Autodesk Inventor part; units mm, degrees
ref_plane "YZ Plane" through (0, 0, 0) normal (1, 0, 0) x (0, 1, 0)
ref_plane "XZ Plane" through (0, 0, 0) normal (0, 1, 0) x (-1, 0, 0)
ref_plane "XY Plane" through (0, 0, 0) normal (0, 0, 1) x (1, 0, 0)
sketch "Sketch1" plane through (0, 0, 0) normal (0, 0, 1) x (1, 0, 0)
  line L0 (-4.5, -2.26) -> (4.5, -2.26)
  line L1 (4.5, -2.26) -> (4.5, 2.26)
  line L2 (4.5, 2.26) -> (-4.5, 2.26)
  line L3 (-4.5, 2.26) -> (-4.5, -2.26)
  line L4 (-4.5, -2.26) -> (4.5, 2.26) construction
  line L5 (4.5, -2.26) -> (-4.5, 2.26) construction
  point P0 (0, 0)
  dimension "d0" = 9
  dimension "d1" = 4.52
extrude "Extrusion1" add sketch "Sketch1" along normal blind 2.5
sketch "Sketch2" plane through (0, 0, 0) normal (0, 0, 1) x (1, 0, 0)
  line L0 (-6, -5) -> (6, -5)
  line L1 (6, -5) -> (6, 5)
  line L2 (6, 5) -> (-6, 5)
  line L3 (-6, 5) -> (-6, -5)
  line L4 (-6, -5) -> (6, 5) construction
  line L5 (6, -5) -> (-6, 5) construction
  point P0 (0, 0)
  dimension "d4" = 12
  dimension "d5" = 10
extrude "Extrusion2" add sketch "Sketch2" against normal blind 20
fillet "Fillet1" radius 2 4 edges at (-6, 5, -10) (6, 5, -10) (6, -5, -10) (-6, -5, -10)
sketch "Sketch3" plane through (0, 0, 0) normal (0, 0, 1) x (1, 0, 0)
  line L0 (-9, 0) -> (9, 0) construction
  circle A0 centre (-9, 0) radius 4.05
  circle A1 centre (9, 0) radius 4.05
  line L1 (-9, 4.05) -> (9, 4.05)
  line L2 (9, 4.05) -> (9, -4.05)
  line L3 (9, -4.05) -> (-9, -4.05)
  line L4 (-9, -4.05) -> (-9, 4.05)
  point P0 (0, 0)
  point P1 (0, 0)
  dimension "d10" = 8.1
  dimension "d9" = 18
extrude "Extrusion3" add sketch "Sketch3" against normal blind 5.2
hole "Hole1" at (-9, 0, 0) at (9, 0, 0) direction (0, 0, -1) diameter 2.459 end through all
fillet "Fillet2" radius 0.5 4 edges at (-4.5, 2.26, 1.25) (4.5, 2.26, 1.25) (4.5, -2.26, 1.25) (-4.5, -2.26, 1.25)
properties part number "103367_Panel_Side_USB"
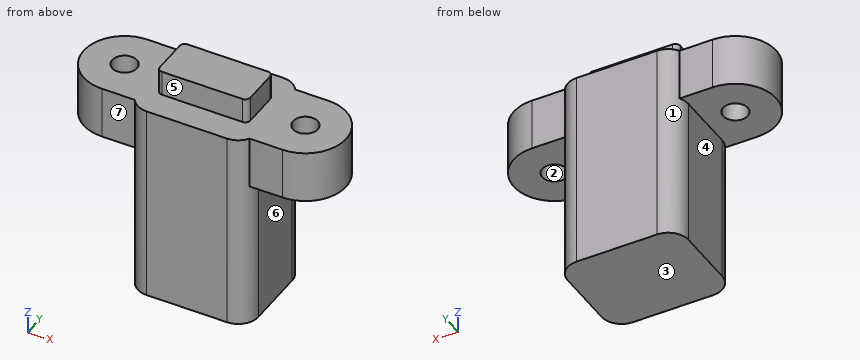
Geometry: final body of the model. Coordinates: model frame, mm. Face numbers are marked on the shaded views. A direction names the side the tool comes from. Give positions to 0.01 mm unless a question says otherwise; leave off trailing zeros. Write each loop counter-clockwise with the first axis right and the second up, starting at its lowest first coordinate (ties: lowest second). Pieces come first, ordered by that corner, then holes.
(1) Mould query, pull axis Y, two halves, no side actions, for the marked faces 1, 2 and 3. Classes: released by +Y, released by -Y, zero draft, split by the parting line, or undercut.
(2) Cut plane B-B, the plane y = 0. Return loops of the section in (x, z).
(3) First-contact query: P1, Ø6, axis at x = 11, y = 1, coming from the -Z side; P2, Ø3, axis at x = -10.5, z = -0.5, coming from the -Y side; P3, Ø3, axis at x = 9, y = 0, coming from the +Z side. Flat tips, straight axial feed; report the tip coordinate or a pass-through.
(4) Ray query, line 1 (X direction, y = 0, z = -1.9); line 2 (Y direction, x = 9, z = -2.4); line 3 (Z direction, x = 8.5, y = 1.25). Return the intervals inside material, ascending.
(5) Access query for the marked faces 4, 5, 6 and 7. Directions: +Z, -Z, +X, -X, +Y, -Y. A direction counts if a zero-diameter tool reaches every point of the face in a straight line with its end or side. Return the directions, or none.
(6) Cut plane D-D, the plane z = -11.5. Return loops of the section in (x, y), then the cut area to 3 significant figures.
(7) Cut plane A-A, the plane z = -3.75. Return loops of the section in (x, y).
(8) Cut plane C-C, the plane x = 0.5. Return loops of the section in (y, z), then the cut area to 3 significant figures.
Values follow:
1. face 1: released by +Y
1. face 2: undercut
1. face 3: zero draft
2. outline: (-13.05, -5.2) - (-10.23, -5.2) - (-10.23, 0) - (-13.05, 0) - close; (-7.77, -5.2) - (-6, -5.2) - (-6, -20) - (6, -20) - (6, -5.2) - (7.77, -5.2) - (7.77, 0) - (4.5, 0) - (4.5, 2.5) - (-4.5, 2.5) - (-4.5, 0) - (-7.77, 0) - close; (10.23, -5.2) - (13.05, -5.2) - (13.05, 0) - (10.23, 0) - close
3. P1: stops at z = -5.2
3. P2: stops at y = -4.05
3. P3: stops at z = 0
4. line 1: x = -13.05 to -10.23, -7.77 to 7.77, 10.23 to 13.05
4. line 2: y = -4.05 to -1.23, 1.23 to 4.05
4. line 3: z = -5.2 to 0
5. face 4: -Z, -X, +Y, -Y
5. face 5: +Z, +X, -X, -Y
5. face 6: -Z, +X, +Y, -Y
5. face 7: +Z, -Z, -X, -Y
6. outline: (-6, -3) arc R2 ccw to (-4, -5) - (4, -5) arc R2 ccw to (6, -3) - (6, 3) arc R2 ccw to (4, 5) - (-4, 5) arc R2 ccw to (-6, 3) - close
6. area: 117 mm2
7. outline: (-9, -4.05) - (-5.7, -4.05) arc R2 ccw to (-4, -5) - (4, -5) arc R2 ccw to (5.7, -4.05) - (9, -4.05) arc R4.05 ccw to (9, 4.05) - (5.7, 4.05) arc R2 ccw to (4, 5) - (-4, 5) arc R2 ccw to (-5.7, 4.05) - (-9, 4.05) arc R4.05 ccw to start; hole circle Ø2.46 at (-9, 0); hole circle Ø2.46 at (9, 0)
8. outline: (-5, -20) - (5, -20) - (5, 0) - (2.26, 0) - (2.26, 2.5) - (-2.26, 2.5) - (-2.26, 0) - (-5, 0) - close
8. area: 211 mm2
